from build123d import *
from build123d.topology import SkipClean

# Parameters (mm, degrees)
SKETCH_1_W               = 34.5
SKETCH_1_H               = 96.8
SKETCH_3_R               = 1.5
CUT_EXTRUDE_1_DEPTH      = 102.634147805
PATTERN_CIRCULAR_1_COUNT = 4
EXTRUDE_2_DEPTH          = 5
EXTRUDE_3_DEPTH          = 5
SKETCH_4_R               = 2
CUT_EXTRUDE_2_DEPTH      = 8


with BuildPart() as part:
    # 草图1 → 旋转1 (revolve)
    with SkipClean():  # the faces are left unmerged after this step: merging them gives an invalid solid
        with BuildSketch(Plane.XY, mode=Mode.PRIVATE) as revolve_1_sk:
            with Locations((42.25, 0)):
                Rectangle(SKETCH_1_W, SKETCH_1_H)
            Polygon((-25, 57), (-37.5, 57), (-37.5, 49), (-32.5, 49), (-32.5, 48.4), (-59.5, 48.4), (-59.5, -48.4), (-25, -48.4), align=None)
        revolve(revolve_1_sk.sketch.rotate(Axis((0, 57, 0), (0, -1, 0)), 180), axis=Axis((0, 57, 0), (0, -1, 0)))

    # 草图3 → 切除-拉伸1 (cut, through all)
    with SkipClean():  # the faces are left unmerged after this step: merging them gives an invalid solid
        with BuildSketch(Plane.XY):
            with Locations((0, 54)):
                Circle(SKETCH_3_R)
        cut_extrude_1 = extrude(amount=-CUT_EXTRUDE_1_DEPTH, mode=Mode.SUBTRACT)

    # 阵列(圆周)1: 切除-拉伸1 ×4 about axis
    with SkipClean():  # the faces are left unmerged after this step: merging them gives an invalid solid
        pattern_circular_1_axis = Axis((0, 57, 0), (0, 1, 0))
        for i in range(1, PATTERN_CIRCULAR_1_COUNT):
            add(cut_extrude_1.rotate(pattern_circular_1_axis, i * 360 / PATTERN_CIRCULAR_1_COUNT), mode=Mode.SUBTRACT)

    # 草图5 → 凸台-拉伸2 (add)
    with SkipClean():  # the faces are left unmerged after this step: merging them gives an invalid solid
        with BuildSketch(Plane(origin=(0, 57, 0), x_dir=(1, 0, 0), z_dir=(0, 1, 0))):
            with BuildLine():
                ThreePointArc((14.592688862, 26.554536934), (21.42533547, 21.42533547), (26.554536934, 14.592688862))
                ThreePointArc((26.554536934, 14.592688862), (25.764976005, 11.876700361), (23.048987504, 12.66626129))
                ThreePointArc((23.048987504, 12.66626129), (18.596908345, 18.596908345), (12.66626129, 23.048987504))
                ThreePointArc((12.66626129, 23.048987504), (11.876700361, 25.764976005), (14.592688862, 26.554536934))
            make_face()
            with BuildLine():
                ThreePointArc((-26.554536934, -14.592688862), (-25.764976005, -11.876700361), (-23.048987504, -12.66626129))
                ThreePointArc((-23.048987504, -12.66626129), (-18.596908345, -18.596908345), (-12.66626129, -23.048987504))
                ThreePointArc((-12.66626129, -23.048987504), (-11.876700361, -25.764976005), (-14.592688862, -26.554536934))
                ThreePointArc((-14.592688862, -26.554536934), (-21.42533547, -21.42533547), (-26.554536934, -14.592688862))
            make_face()
            with BuildLine():
                ThreePointArc((-14.592688862, 26.554536934), (-11.876700361, 25.764976005), (-12.66626129, 23.048987504))
                ThreePointArc((-12.66626129, 23.048987504), (-18.596908345, 18.596908345), (-23.048987504, 12.66626129))
                ThreePointArc((-23.048987504, 12.66626129), (-25.764976005, 11.876700361), (-26.554536934, 14.592688862))
                ThreePointArc((-26.554536934, 14.592688862), (-21.42533547, 21.42533547), (-14.592688862, 26.554536934))
            make_face()
        extrude(amount=EXTRUDE_2_DEPTH)

    # 草图6 → 凸台-拉伸3 (add)
    with SkipClean():  # the faces are left unmerged after this step: merging them gives an invalid solid
        with BuildSketch(Plane.XZ.offset(48.4)):
            with BuildLine():
                Line((43.716333699, 29.281088913), (47.216333699, 23.218911087))
                ThreePointArc((47.216333699, 23.218911087), (45.935244785, 18.437822174), (41.154155872, 19.718911087))
                Line((41.154155872, 19.718911087), (37.654155872, 25.781088913))
                ThreePointArc((37.654155872, 25.781088913), (38.935244785, 30.562177826), (43.716333699, 29.281088913))
            make_face()
            with BuildLine():
                Line((43.716333699, -29.281088913), (47.216333699, -23.218911087))
                ThreePointArc((47.216333699, -23.218911087), (45.935244785, -18.437822174), (41.154155872, -19.718911087))
                Line((41.154155872, -19.718911087), (37.654155872, -25.781088913))
                ThreePointArc((37.654155872, -25.781088913), (38.935244785, -30.562177826), (43.716333699, -29.281088913))
            make_face()
            with BuildLine():
                Line((-43.716333699, -29.281088913), (-47.216333699, -23.218911087))
                ThreePointArc((-47.216333699, -23.218911087), (-45.935244785, -18.437822174), (-41.154155872, -19.718911087))
                Line((-41.154155872, -19.718911087), (-37.654155872, -25.781088913))
                ThreePointArc((-37.654155872, -25.781088913), (-38.935244785, -30.562177826), (-43.716333699, -29.281088913))
            make_face()
            with BuildLine():
                Line((-43.716333699, 29.281088913), (-47.216333699, 23.218911087))
                ThreePointArc((-47.216333699, 23.218911087), (-45.935244785, 18.437822174), (-41.154155872, 19.718911087))
                Line((-41.154155872, 19.718911087), (-37.654155872, 25.781088913))
                ThreePointArc((-37.654155872, 25.781088913), (-38.935244785, 30.562177826), (-43.716333699, 29.281088913))
            make_face()
        extrude(amount=EXTRUDE_3_DEPTH)

    # 草图4 → 切除-拉伸2 (cut)
    with SkipClean():  # the faces are left unmerged after this step: merging them gives an invalid solid
        with BuildSketch(Plane.XZ.offset(48.4)):
            with Locations((-6.25, 51.75)):
                Circle(SKETCH_4_R)
            with Locations(Location((6.25, 51.75, 0), (0, 0, 180))):
                Circle(SKETCH_4_R)
            with Locations(Location((-6.25, -51.75, 0), (0, 0, 180))):
                Circle(SKETCH_4_R)
            with Locations((6.25, -51.75)):
                Circle(SKETCH_4_R)
        extrude(amount=-CUT_EXTRUDE_2_DEPTH, mode=Mode.SUBTRACT)


solid = part.part
Read the model definition and answer for the solid it produces. Units are mm, in the model's axes. A direction names the side the tool comes from. Round coordinates to 2 decimals unless told otherwise and drop trailing zeros. Order: outer loops, then holes, each group sorted by start corner. A loop starts at its lowest first (then second) coordinate and runs counter-clockwise, first axis right, second up.
1) The part is cut by section B-B on y = 42. Write down the section's boundary in (x, z).
2) Flat-ended cylindrical pins translate along their axes: pin 1 (3 mm diameter, centred on x = -7, z = -52.5, fed in from -Y); pin 2 (10 mm diameter, centred on y = 37, z = 13, fed in from +X); pin 3 (5 mm diameter, centred on x = 0, y = 54, fed in from +Z). Find the tip coordinate at first contact, or state that the pin passes through.
3) The part is cut by section D-D on z = 51.75. Write down the section's boundary in (x, y).
4) Straight lines are drawn through the part: L1, parallel to Y at x = -16.5, z = 32; L2, parallel to Z at x = 6.25, y = -42; L3, parallel to X at y = -41, z = 50. For each, find the intervals that lie inside material, in ascending order.
5) The part is cut by section A-A on x = 34.5. Write down the section's boundary in (y, z).
6) The mould has two halves that part along X. Classify faces 5 (the face through (17.3, 52.94, -33.27)), 6 (the face through (45.442, -50.865, 26.292)), 7 (the face through (-45.442, -50.865, -26.292)), 8 (the face through (18.67, 59.465, -18.523)): released by +X, released by -X, zero draft, split by the parting line, or undercut.
7) The part is cut by section C-C on x = -6.25. Write down the section's boundary in (y, z).
8) For faces 1 (the face through (-5.327, -44.456, 49.976)), 2 (the face through (-18.67, 59.465, 18.523)), 3 (the face through (43, -53.4, 25)), 4 (the face through (-11.898, 59.465, -25.803)), determine the directions among +Z, -Z, +X, -X, +Y, -Y from which every point of the face is accessible in a straight line to the end or side of a thin tool.
Resolved:
1. outline: circle Ø119 at (0, 0); hole circle Ø50 at (0, 0)
2. pin 1: stops at y = -48.4
2. pin 2: stops at x = 58.96
2. pin 3: stops at z = 37.5
3. outline: (-29.36, -48.4) - (-8.25, -48.4) - (-8.25, -40.4) - (-4.25, -40.4) - (-4.25, -48.4) - (4.25, -48.4) - (4.25, -40.4) - (8.25, -40.4) - (8.25, -48.4) - (29.36, -48.4) - (29.36, 48.4) - (-29.36, 48.4) - close
4. L1: y = -48.4 to 48.4, 49 to 57
4. L2: z = -59.17 to -53.75, -49.75 to -24.21, 24.21 to 49.75, 53.75 to 59.17
4. L3: x = -32.25 to -7.22, -5.28 to 5.28, 7.22 to 32.25
5. outline: (-48.4, -48.48) - (48.4, -48.48) - (48.4, 48.48) - (-48.4, 48.48) - close; (49, -14.7) - (57, -14.7) - (57, 14.7) - (49, 14.7) - close; hole circle Ø3 at (54, 0)
6. face 5: split by the parting line
6. face 6: released by +X
6. face 7: released by -X
6. face 8: undercut
7. outline: (-48.4, -59.17) - (48.4, -59.17) - (48.4, -31.89) - (49, -31.89) - (49, -36.98) - (57, -36.98) - (57, -24.21) - (-48.4, -24.21) - (-48.4, -49.75) - (-40.4, -49.75) - (-40.4, -53.75) - (-48.4, -53.75) - close; (-48.4, 24.21) - (57, 24.21) - (57, 36.98) - (49, 36.98) - (49, 31.89) - (48.4, 31.89) - (48.4, 59.17) - (-48.4, 59.17) - (-48.4, 53.75) - (-40.4, 53.75) - (-40.4, 49.75) - (-48.4, 49.75) - close
8. face 1: -Y
8. face 2: +X, +Y
8. face 3: +Z, -Z, +X, -X, -Y
8. face 4: +Y
